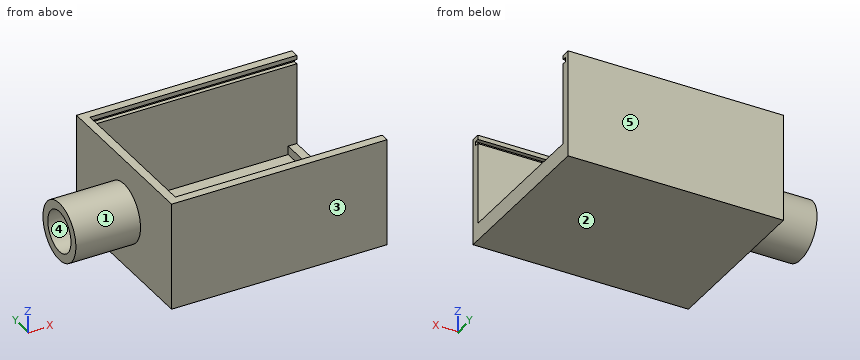
Autodesk Fusion 360 part; units mm, degrees
sketch "Sketch1" plane through (0, 0, 0) normal (0, 0, 1) x (1, 0, 0)
  line L0 (0, 0) -> (50, 0)
  line L1 (50, 0) -> (50, 39)
  line L2 (50, 39) -> (0, 39)
  line L3 (0, 39) -> (0, 0)
  line L4 (2, 2) -> (48, 2)
  line L5 (48, 2) -> (48, 37)
  line L6 (48, 37) -> (2, 37)
  line L7 (2, 37) -> (2, 2)
  dimension "d1" = 46
  dimension "d2" = 2
  dimension "d3" = 2
  dimension "d4" = 2
  dimension "d5" = 2
  dimension "d6" = 35
extrude "Extrude1" add sketch "Sketch1" along normal blind 2 contours L4 L5 L6 L7
extrude "Extrude2" add sketch "Sketch1" along normal blind 25
sketch "Sketch2" plane through (50, 0, 0) normal (1, 0, 0) x (0, 1, 0)
  line L0 (0, 0) -> (39, 0)
  line L1 (39, 0) -> (39, 25)
  line L2 (39, 25) -> (0, 25)
  line L3 (0, 25) -> (0, 0)
  line L4 (2, 25) -> (2, 24)
  line L5 (2, 24) -> (1, 24)
  line L6 (1, 24) -> (1, 23)
  line L7 (1, 23) -> (38, 23)
  line L8 (38, 23) -> (38, 24)
  line L9 (38, 24) -> (37, 24)
  line L10 (37, 24) -> (37, 25)
  line L11 (2, 23) -> (37, 23)
  line L12 (37, 23) -> (37, 4)
  line L13 (37, 4) -> (2, 4)
  line L14 (2, 4) -> (2, 23)
  dimension "d11" = 1
  dimension "d12" = 1
  dimension "d13" = 1
  dimension "d14" = 1
  dimension "d15" = 1
  dimension "d16" = 1
  dimension "d17" = 1
  dimension "d18" = 19
extrude "Extrude3" cut sketch "Sketch2" against normal up to surface (48 mm away) contours L2 L4 L5 L6 L7 L8 L9 L10 L11 | L7 L11 L12 L13 L14
sketch "Sketch3" plane through (0, 0, 0) normal (-1, 0, 0) x (0, -1, 0)
  line L0 (-39, 0) -> (0, 0)
  line L1 (0, 0) -> (0, 25)
  line L2 (0, 25) -> (-39, 25)
  line L3 (-39, 25) -> (-39, 0)
  circle A0 centre (-19.5, 12.5) radius 6.75
  circle A1 centre (-19.5, 12.5) radius 4.75
  point P0 (-19.5, 25)
  point P1 (0, 12.5)
  dimension "d21" = 2
  dimension "d22" = 9.5
extrude "Extrude4" add sketch "Sketch3" along normal blind 15 contours A0
Here's how the part is built. I have some questions about the finished solid (model axes, mm). Face numbers are marked on the shaded views. A direction names the side the tool comes from. Give positions to 0.01 mm unless a question says otherwise; leave off trailing zeros. Order: outer loops, then holes, each group sorted by start corner. A loop starts at its lowest first (then second) coordinate and runs counter-clockwise, first axis right, second up. Notation, with made-up numbers: M 42.25,26 L 96.25,26 A9 ccw 96.25,37 Z; hole C 32,37 d4. An arc over 180 degrees is marked long. Use a Markdown table: item, result. Add a question column.
1. For pin 1 Ø5 at (y, z) = (21.5, 13) entering from -X; pin 2 Ø11 at (y, z) = (19.5, 12.5) entering from -X; pin 3 Ø3 at (y, z) = (4.5, 22.5) entering from +X; pin 4 Ø1 at (x, y) = (49, 25) entering from +Z, each with a flat end and sliding along its axis, tell me the tip position at first contact or that it passes through.
2. Suppose I cut it at C-C (x = 8.5). List the corners of the cut face in (y, z) for me.
3. If we mould it in two halves opening along Y, with no side actions, what happens to the marked faces 3, 4 and 5? For each: +Y half, -Y half, draft (parallel to the pull), parting line (faces both ways), or undercut.
4. I need wall thicknesses on probe 1 along X at (y, z) = (24.5, 3.75); probe 2 along Y at (x, z) = (40.5, 20.75); probe 3 along Z at (x, y) = (-10.75, 19.5). Which ranges of each line are inside material? Lowest first, please. Write a range as from..to.
5. On a 3-axis mill with a long thin cutter (end or side, diameter ignored), from which of +Z, -Z, +X, -X, +Y, -Y can I reach the whole of each face in a straight line? I mean the marked faces 1 and 2. Say none if no direction works.
6. Suppose I cut it at D-D (x = -8). List the corners of the cut face in (y, z) for me, and give its area (3 significant figures).
7. Suppose I cut it at B-B (z = 12.5). List the corners of the cut face in (x, y) for me.
8. Suppose I cut it at A-A (y = 34.5). List the corners of the cut face in (x, z) for me, and give its area (3 significant figures).
Results list:
| question | item | result |
|---|---|---|
| 1 | pin 1 | stops at x = 0 |
| 1 | pin 2 | stops at x = -15 |
| 1 | pin 3 | stops at x = 2 |
| 1 | pin 4 | stops at z = 4 |
| 2 | outline | M 0,0 L 39,0 L 39,25 L 37,25 L 37,24 L 38,24 L 38,23 L 37,23 L 37,2 L 2,2 L 2,23 L 1,23 L 1,24 L 2,24 L 2,25 L 0,25 Z |
| 3 | face 3 | -Y half |
| 3 | face 4 | undercut |
| 3 | face 5 | +Y half |
| 4 | probe 1 | x = 0..2, 48..50 |
| 4 | probe 2 | y = 0..2, 37..39 |
| 4 | probe 3 | z = 5.75..7.75, 17.25..19.25 |
| 5 | face 1 | -X |
| 5 | face 2 | -Z, +X, -X, +Y, -Y |
| 6 | outline | C 19.5,12.5 d13.5; hole C 19.5,12.5 d9.5 |
| 6 | area | 72.3 mm² |
| 7 | outline | M -15,12.75 L 0,12.75 L 0,0 L 50,0 L 50,2 L 2,2 L 2,37 L 50,37 L 50,39 L 0,39 L 0,26.25 L -15,26.25 L -15,24.25 L 0,24.25 L 0,14.75 L -15,14.75 Z |
| 8 | outline | M 0,0 L 50,0 L 50,4 L 48,4 L 48,2 L 2,2 L 2,25 L 0,25 Z |
| 8 | area | 150 mm² |
